Autodesk Inventor part; units mm, degrees
ref_plane "YZ Plane" through (0, 0, 0) normal (1, 0, 0) x (0, 1, 0)
ref_plane "XZ Plane" through (0, 0, 0) normal (0, 1, 0) x (-1, 0, 0)
ref_plane "XY Plane" through (0, 0, 0) normal (0, 0, 1) x (1, 0, 0)
sketch "スケッチ1" plane through (0, 0, 0) normal (0, 0, 1) x (1, 0, 0)
  line L0 (-55, -95) -> (55, -95)
  line L1 (55, -95) -> (55, 95)
  line L2 (55, 95) -> (-55, 95)
  line L3 (-55, 95) -> (-55, -95)
  line L4 (-55, -95) -> (55, 95) construction
  line L5 (55, -95) -> (-55, 95) construction
  circle A0 centre (0, 40) radius 6.5
  line L6 (0, 40) -> (-55, 95)
  point P0 (0, 0)
  dimension "d0" = 110
  dimension "d39" = 45
extrude "プレート1" add sketch "スケッチ1" along normal blind 2 contours L3 L2 L1 L0 | A0
sketch "スケッチ2" plane through (0, 0, 2) normal (0, 0, 1) x (1, 0, 0)
  circle A0 centre (0, -40) radius 12.5
  point P0 (0, 0)
  point P1 (0, -27.5)
  point P2 (-12.5, -40)
  point P3 (0, -52.5)
  point P4 (12.5, -40)
  dimension "d8" = 25
  dimension "d11" = 360
hole "穴1" at (0, -27.5, 2) at (-12.5, -40, 2) at (0, -52.5, 2) at (12.5, -40, 2) direction (0, 0, -1) diameter 3.2 end through all
sketch "スケッチ3" plane through (0, 0, 2) normal (0, 0, 1) x (1, 0, 0)
  circle A0 centre (0, 38.4) radius 10
  point P0 (0, 0)
  dimension "d22" = 20
  dimension "d58" = 38.4
extrude "押し出し1" cut sketch "スケッチ3" against normal blind 10
sketch "スケッチ4" plane through (0, 0, 2) normal (0, 0, 1) x (1, 0, 0)
  line L0 (-55, 95) -> (55, 95)
  line L1 (-55, -95) -> (-55, 95)
  line L2 (55, 95) -> (55, -95)
  line L3 (55, -95) -> (-55, -95)
  line L4 (50, 90) -> (-50, 90)
  line L5 (-50, 90) -> (-50, -90)
  line L6 (-50, -90) -> (50, -90)
  line L7 (50, -90) -> (50, 90)
  point P0 (0, 0)
  point P1 (-50, 0)
  point P2 (50, 0)
  dimension "d25" = 5
hole "穴2" at (-50, 90, 2) at (50, 90, 2) at (50, -90, 2) at (-50, -90, 2) at (50, 0, 2) at (-50, 0, 2) direction (0, 0, -1) diameter 4.3 end through all
fillet "コーナーR1" radius 5 4 edges at (55, 95, 1) (-55, 95, 1) (-55, -95, 1) (55, -95, 1)
sketch "スケッチ5" plane through (0, 0, 2) normal (0, 0, 1) x (1, 0, 0)
  circle A0 centre (0, -38.4) radius 41
  point P0 (0, 0)
  dimension "d35" = 82
  dimension "d59" = 38.4
extrude "押し出し2" cut sketch "スケッチ5" against normal blind 10
sketch "スケッチ6" plane through (0, 0, 2) normal (0, 0, 1) x (1, 0, 0)
  circle A0 centre (0, -38.4) radius 41
  circle A1 centre (0, -38.4) radius 53.5
  circle A2 centre (0, 38.4) radius 10
  circle A3 centre (0, 38.4) radius 20
  point P0 (0, 0)
  point P1 (-46.3324, -65.15)
  point P2 (-26.75, -84.7324)
  point P3 (0, -91.9)
  point P4 (26.75, -84.7324)
  point P5 (46.3324, -65.15)
  point P6 (53.5, -38.4)
  point P7 (46.3324, -11.65)
  point P8 (26.75, 7.9324)
  point P9 (0, 15.1)
  point P10 (-26.75, 7.9324)
  point P11 (-46.3324, -11.65)
  point P12 (-53.5, -38.4)
  point P13 (-10, 55.7205)
  point P14 (-20, 38.4)
  point P15 (-10, 21.0795)
  point P16 (10, 21.0795)
  point P17 (20, 38.4)
  point P18 (10, 55.7205)
  dimension "d40" = 107
  dimension "d52" = 40
  dimension "d43" = 360
  dimension "d55" = 360
  dimension "d57" = 0
hole "穴3" at (-26.75, -84.7324, 2) at (-46.3324, -65.15, 2) at (-46.3324, -11.65, 2) at (-26.75, 7.9324, 2) at (26.75, 7.9324, 2) at (46.3324, -11.65, 2) at (46.3324, -65.15, 2) at (26.75, -84.7324, 2) at (10, 55.7205, 2) at (20, 38.4, 2) at (-20, 38.4, 2) at (-10, 55.7205, 2) at (0, 15.1, 2) at (10, 21.0795, 2) at (-10, 21.0795, 2) direction (0, 0, -1) diameter 3.2 end through all
equation "\"d20\" = Thickness"
equation "\"d50\" = Thickness"
equation "\"d2\" = Thickness"
equation "\"BendRadius\" = Thickness"
equation "\"BendReliefWidth\" = Thickness"
equation "\"BendReliefDepth\" = 0.5 * Thickness"
equation "\"CornerReliefSize\" = 4 * Thickness"
equation "\"MinimumRemnant\" = 2 * Thickness"
equation "\"TransitionRadius\" = BendRadius"
equation "\"JacobiRadiusSize\" = BendRadius"
equation "\"GapSize\" = Thickness"
properties part number "carbonplate2" material "CFRP"
The model under review builds one solid part; all positions refer to its coordinate system, in mm. Round coordinates to 2 decimals unless told otherwise and drop trailing zeros. Loops run counter-clockwise (first coordinate to the right, second up) from the corner with the lowest first, then second, coordinate; pieces in that order, holes last. Notation, with made-up numbers: (-16, 70) -> (-10, 70) arc R12 ccw to (-10, 78) -> close; hole circle Ø4 at (70.5, 72). An arc over 180 degrees is marked (long way). One line per question, with ' | ' between items. Start each with the question number.
Item 1: Wall thickness on line 1 along Y through (x, z) = (50, 0.55); line 2 along X through (y, z) = (90, 0.8); line 3 along Y through (x, z) = (0, 1.4): over which ranges is each line inside the solid? List them lowest first. Write a range as [from, to].
Item 2: Draft analysis for pull direction Y (two halves, no side actions). For faces 1 (the face through (-54, -93, 1)), 2 (the face through (-50.09, -87.85, 0.99)), 3 (the face through (54, 93, 1)), state which applies: +Y half, -Y half, draft (parallel to the pull), parting line (faces both ways), or undercut.
Item 3: Add section C-C, the plane z = 0.65. Count the separate pieces of the cut face and the enclosed holes in it, then the cut area to 3 significant figures.
Item 4: Add section A-A, the plane x = -31.5. Write out the cut boundary in (y, z).
Item 5: Add section B-B, the plane y = -74.5. Write out the cut boundary in (x, z).
Return value:
1) line 1: y = [-95, -92.15], [-87.85, -2.15], [2.15, 87.85], [92.15, 95] | line 2: x = [-55, -52.15], [-47.85, 47.85], [52.15, 55] | line 3: y = [-95, -79.4], [2.6, 13.5], [16.7, 28.4], [48.4, 95]
2) face 1: -Y half | face 2: undercut | face 3: +Y half
3) separate pieces: 1 | enclosed holes: 23 | area: 15,100 mm2
4) outline: (-95, 0) -> (-64.64, 0) -> (-64.64, 2) -> (-95, 2) -> close; (-12.16, 0) -> (95, 0) -> (95, 2) -> (-12.16, 2) -> close
5) outline: (-55, 0) -> (-19.44, 0) -> (-19.44, 2) -> (-55, 2) -> close; (19.44, 0) -> (55, 0) -> (55, 2) -> (19.44, 2) -> close
